Check sheet for the modelled part. Datum: model origin and axes. Units: mm. A direction names the side the tool comes from. Give positions to 0.01 mm unless a question says otherwise; leave off trailing zeros. Loops run counter-clockwise (first coordinate to the right, second up) from the corner with the lowest first, then second, coordinate; pieces in that order, holes last. Notation, with made-up numbers: (-38.5, -33.5) -> (-15.5, -33.5) arc R30 cw to (-15.5, -8.5) -> close; hole circle Ø7 at (-5.75, -22.75). An arc over 180 degrees is marked (long way). Answer as CSV lines item,"result". Start each with the question number.
(1) Section check D-D on y = -0.25. Enter the section's corners in (x, z), plus the area to 3 significant figures.
(2) Gauge pin test, flat ends, axial feed: pin 1 Ø12 at (x, y) = (14.51, -10.73) entering from -Z; pin 2 Ø4.5 at (x, y) = (30.5, -9.5) entering from +Z; pin 3 Ø3 at (y, z) = (-21.5, 5.5) entering from -X; pin 4 Ø1 at (x, z) = (4.5, 2) entering from +Y. Record the tip position at first contact, or that the pin passes through.
(3) Release check for a two-part mould opening along X. For faces 3 (the face through (22, -8, 2)), 4 (the face through (23, -24.232, 3)), 5 (the face through (0.809, -11, 4)) record: pulls with the +X half, pulls with the -X half, needs draft (parallel to the pull), parting line crosses it, or undercut.
(4) Access from +Z, -Z, +X, -X, +Y, -Y to the whole of each face (thin tool, end or side, straight path). Record for faces 1 (the face through (33.8, -9.38, 7.01)), 2 (the face through (20.48, -23.49, 7.24)).
(5) Section check A-A on x = 28. Enter the section's corners in (y, z), plus the area to 3 significant figures.
(6) Material ranges on line 1 (Z direction, x = 22.5, y = -10.25); line 2 (X direction, y = -11, z = 0.5); line 3 (Y direction, x = 14, z = 7), recorded low to high. Write a range as from..to.
(7) Section check B-B on z = 1.5. Enter the section's corners in (x, y).
(8) Section check C-C on z = 7. Enter the section's corners in (x, y).
Autodesk Inventor part; units mm, degrees
ref_plane "YZ Plane" through (0, 0, 0) normal (1, 0, 0) x (0, 1, 0)
ref_plane "XZ Plane" through (0, 0, 0) normal (0, 1, 0) x (-1, 0, 0)
ref_plane "XY Plane" through (0, 0, 0) normal (0, 0, 1) x (1, 0, 0)
sketch "Szkic1" plane through (0, 0, 0) normal (0, 0, 1) x (1, 0, 0)
  line L0 (0.8088, 2.7684) -> (35.0088, 2.7684)
  line L1 (35.0088, 2.7684) -> (35.0088, -24.2316)
  line L2 (35.0088, -24.2316) -> (0.8088, -24.2316)
  line L3 (0.8088, -24.2316) -> (0.8088, 2.7684)
  circle A0 centre (14.5088, -10.7316) radius 9.5
  circle A1 centre (29.5088, -10.7316) radius 2
  circle A2 centre (14.5088, -10.7316) radius 7.5
  point P0 (0, 0)
  dimension "d0" = 34.2
  dimension "d1" = 27
  dimension "d2" = 13.5
  dimension "d3" = 20.5
  dimension "d4" = 19
  dimension "d5" = 13.5
  dimension "d7" = 4
  dimension "d11" = 5.5
  dimension "d14" = 13.5
  dimension "d15" = 2
extrude "Wyciągnięcie proste1" add sketch "Szkic1" along normal blind 8 contours L0 L1 L2 L3
extrude "Wyciągnięcie proste2" add sketch "Szkic1" along normal blind 2 contours A0
chamfer "Faza1" distance 0.5 angle 45 1 edges at (5.0088, -10.7316, 8)
chamfer "Faza2" distance 1.5 angle 45 2 edges at (17.9088, 2.7684, 8) (17.9088, -24.2316, 8)
sketch "Szkic2" plane through (0, 0, 8) normal (0, 0, 1) x (1, 0, 0)
  circle A0 centre (29.5088, -10.7316) radius 2
  circle A1 centre (29.5088, -10.7316) radius 4.5
  point P0 (0, 0)
  dimension "d30" = 9
extrude "Wyciągnięcie proste5" cut sketch "Szkic2" against normal blind 2
fillet "Zaokrąglenie1" radius 10 2 edges at (0.8088, -24.2316, 3.25) (0.8088, 2.7684, 3.25)
properties part number "3DP_ABS_Y_Axis_Pulley_Rod_Side_Bearing_Block"
Working result:
1,outline,"(3.65, 0) -> (35.01, 0) -> (35.01, 8) -> (3.65, 8) -> close"
1,area,"251 mm^2"
2,pin 1,"passes through"
2,pin 2,"stops at z = 6"
2,pin 3,"stops at x = 2.64"
2,pin 4,"stops at y = 0.91"
3,face 3,"undercut"
3,face 4,"needs draft"
3,face 5,"pulls with the -X half"
4,face 1,"+Z"
4,face 2,"+Z, +X, -X, -Y"
5,outline,"(-24.23, 0) -> (-12.04, 0) -> (-12.04, 6) -> (-14.97, 6) -> (-14.97, 8) -> (-22.73, 8) -> (-24.23, 6.5) -> close; (-9.42, 0) -> (2.77, 0) -> (2.77, 6.5) -> (1.27, 8) -> (-6.49, 8) -> (-6.49, 6) -> (-9.42, 6) -> close"
5,area,"181 mm^2"
6,line 1,"z = 0..2"
6,line 2,"x = 0.81..7.01, 22..27.53, 31.49..35.01"
6,line 3,"y = -23.73..-20.22, -1.25..2.27"
7,outline,"(0.81, -14.23) arc R10 ccw to (10.81, -24.23) -> (35.01, -24.23) -> (35.01, 2.77) -> (10.81, 2.77) arc R10 ccw to (0.81, -7.23) -> close; hole circle Ø15 at (14.51, -10.73); hole circle Ø4 at (29.51, -10.73)"
8,outline,"(0.81, -14.23) arc R10 ccw to (7.69, -23.73) -> (35.01, -23.73) -> (35.01, 2.27) -> (7.69, 2.27) arc R10 ccw to (0.81, -7.23) -> close; hole circle Ø19 at (14.51, -10.73); hole circle Ø9 at (29.51, -10.73)"
